Source: CAD feature listing. Evaluate the final solid. Frame: model axes, mm. Face numbers are marked on the shaded views. A direction names the side the tool comes from. Coordinates: 2 decimals unless noted, no trailing zeros. Write each loop counter-clockwise with the first axis right and the second up, starting at its lowest first coordinate (ties: lowest second). Pieces come first, ordered by that corner, then holes. Notation, with made-up numbers: (23, -28.5) -> (78, -28.5) arc R21 ccw to (78, -21.5) -> close; hole circle Ø9 at (77, 1). An arc over 180 degrees is marked (long way). One line per item, written item: value. Start each with the question number.
1. Section query A-A, the plane x = 0. Output: boundary loops of the cut face in (y, z), and give its area (3 significant figures).
2. Section query B-B, the plane y = -10. Output: boundary loops of the cut face in (x, z), and give its area (3 significant figures).
3. Section query D-D, the plane y = -19. Output: boundary loops of the cut face in (x, z), and give its area (3 significant figures).
4. Line query: line 1 (Z direction, x = 14, y = -26); line 2 (Y direction, x = -7.75, z = 0.95); line 3 (Y direction, x = 17.5, z = 19). Output: solid intervals per line, ascending.
5. First-contact query: P1, Ø2.5, axis at x = 14.25, z = 33.85, coming from the +Y side; P2, Ø4, axis at x = 7.75, y = -13.42, coming from the +Z side; P3, Ø4, axis at x = -14.25, z = 33.85, coming from the +Y side; P4, Ø3.5, axis at y = 3.5, z = 1, coming from the -X side. Flat tips, straight axial feed; report the tip coordinate or a pass-through.
6. Access query for the marked faces 1 and 2. Directions: +Z, -Z, +X, -X, +Y, -Y. A direction counts if a zero-diameter tool reaches every point of the face in a straight line with its end or side. Return the directions, or none.
7. Section query C-C, the plane z = 11.35. Output: boundary loops of the cut face in (x, y).
from build123d import *

# Parameters (mm, degrees)
ESBO_O1_R                = 1.5
RESSALTO_EXTRUS_O1_DEPTH = 3
ESBO_O2_W                = 40
ESBO_O2_H                = 42.2
ESBO_O2_R                = 1.5
RESSALTO_EXTRUS_O2_DEPTH = 3


with BuildPart() as part:
    # Esboço1 → Ressalto-extrusão1 (new body)
    with BuildSketch(Plane.XY):
        with BuildLine():
            Line((-20, 0), (-20, -28))
            Line((-20, -28), (20, -28))
            Line((20, -28), (20, 0))
            ThreePointArc((20, 0), (0, 20), (-20, 0))
        make_face()
        with Locations((-15.5, 0)):
            Circle(ESBO_O1_R, mode=Mode.SUBTRACT)
        with Locations((-7.75, 13.423393759)):
            Circle(ESBO_O1_R, mode=Mode.SUBTRACT)
        with Locations((7.75, 13.423393759)):
            Circle(ESBO_O1_R, mode=Mode.SUBTRACT)
        with Locations((15.5, 0)):
            Circle(ESBO_O1_R, mode=Mode.SUBTRACT)
        with Locations((7.75, -13.423393759)):
            Circle(ESBO_O1_R, mode=Mode.SUBTRACT)
        with Locations((-7.75, -13.423393759)):
            Circle(ESBO_O1_R, mode=Mode.SUBTRACT)
        with BuildLine():
            Line((6.5, 7.5), (6.5, -7.5))
            ThreePointArc((6.5, -7.5), (0, -14), (-6.5, -7.5))
            Line((-6.5, -7.5), (-6.5, 7.5))
            ThreePointArc((-6.5, 7.5), (0, 14), (6.5, 7.5))
        make_face(mode=Mode.SUBTRACT)
    extrude(amount=RESSALTO_EXTRUS_O1_DEPTH)

    # Esboço2 → Ressalto-extrusão2 (add)
    with BuildSketch(Plane.XZ.offset(28)):
        with Locations((0, 21.1)):
            Rectangle(ESBO_O2_W, ESBO_O2_H)
        with Locations((-14.25, 11.35)):
            Circle(ESBO_O2_R, mode=Mode.SUBTRACT)
        with Locations((14.25, 11.35)):
            Circle(ESBO_O2_R, mode=Mode.SUBTRACT)
        with Locations((14.25, 33.85)):
            Circle(ESBO_O2_R, mode=Mode.SUBTRACT)
        with Locations((-14.25, 33.85)):
            Circle(ESBO_O2_R, mode=Mode.SUBTRACT)
    extrude(amount=-RESSALTO_EXTRUS_O2_DEPTH)


solid = part.part
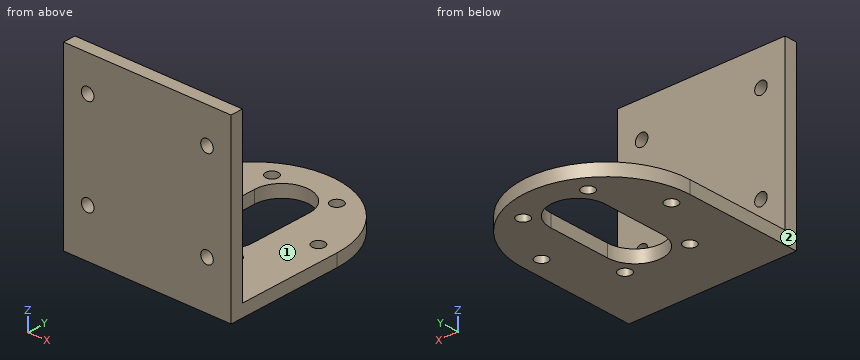
Computed values:
1. outline: (-28, 0) -> (-14, 0) -> (-14, 3) -> (-25, 3) -> (-25, 42.2) -> (-28, 42.2) -> close; (14, 0) -> (20, 0) -> (20, 3) -> (14, 3) -> close
1. area: 178 mm²
2. outline: (-20, 0) -> (-6, 0) -> (-6, 3) -> (-20, 3) -> close; (6, 0) -> (20, 0) -> (20, 3) -> (6, 3) -> close
2. area: 84.0 mm²
3. outline: (-20, 0) -> (20, 0) -> (20, 3) -> (-20, 3) -> close
3. area: 120 mm²
4. line 1: z = 0 to 9.87, 12.83 to 32.37, 35.33 to 42.2
4. line 2: y = -28 to -14.92, -11.92 to 11.92, 14.92 to 18.44
4. line 3: y = -28 to -25
5. P1: passes through
5. P2: stops at z = 3
5. P3: stops at y = -25
5. P4: stops at x = -19.92
6. face 1: +Z, +X, -X, +Y
6. face 2: +Z, -Z, -X, +Y, -Y
7. outline: (-20, -28) -> (-15.75, -28) -> (-15.75, -25) -> (-20, -25) -> close; (-12.75, -28) -> (12.75, -28) -> (12.75, -25) -> (-12.75, -25) -> close; (15.75, -28) -> (20, -28) -> (20, -25) -> (15.75, -25) -> close
